Autodesk Inventor part; units mm, degrees
ref_plane "YZ Plane" through (0, 0, 0) normal (1, 0, 0) x (0, 1, 0)
ref_plane "XZ Plane" through (0, 0, 0) normal (0, 1, 0) x (-1, 0, 0)
ref_plane "XY Plane" through (0, 0, 0) normal (0, 0, 1) x (1, 0, 0)
sketch "Sketch1" plane through (0, 0, 0) normal (0, 0, 1) x (1, 0, 0)
  line L0 (29.994, -18.6437) -> (-29.994, -18.6437)
  line L1 (-29.994, 18.6437) -> (29.994, 18.6437)
  line L2 (29.994, -18.6437) -> (-29.994, 18.6437) construction
  line L3 (-29.994, -18.6437) -> (29.994, 18.6437) construction
  line L4 (29.994, -18.6437) -> (-29.994, -18.6437)
  line L5 (-29.994, -18.6437) -> (-29.994, -17.0588)
  line L6 (-29.994, -17.0588) -> (29.994, -17.0588)
  line L7 (29.994, -17.0588) -> (29.994, -18.6437)
  line L8 (-29.994, 18.6437) -> (-29.994, -17.0588)
  line L9 (29.994, 18.6437) -> (29.994, -17.0588)
  point P0 (0, 0)
extrude "Extrusion1" add sketch "Sketch1" against normal blind 1.5875 contours L6 L8 L1 L9
extrude "Extrusion2" add sketch "Sketch1" along normal blind 11.9062 and the other way blind 1.5875 contours L0 L5 L6 L7
sketch "Sketch2" plane through (-29.994, -17.0588, 0) normal (0, 1, 0) x (1, 0, 0)
  circle A0 centre (4.7625, -5.9531) radius 2.1855
  circle A1 centre (55.5625, -5.9531) radius 2.1855
  point P0 (29.994, 0)
  point P1 (0, 0)
sketch "Sketch3" plane through (0, 0, 0) normal (0, 0, 1) x (1, 0, 0)
  circle A0 centre (-15.2797, 0) radius 2.7871
  circle A1 centre (15.2797, 0) radius 2.7871
extrude "Extrusion3" cut sketch "Sketch3" against normal blind 25.4
extrude "Extrusion4" cut sketch "Sketch2" against normal blind 25.4
fillet "Fillet1" radius 1.5875 1 edges at (0, -18.6437, -1.5875)
properties part number "balun_support"
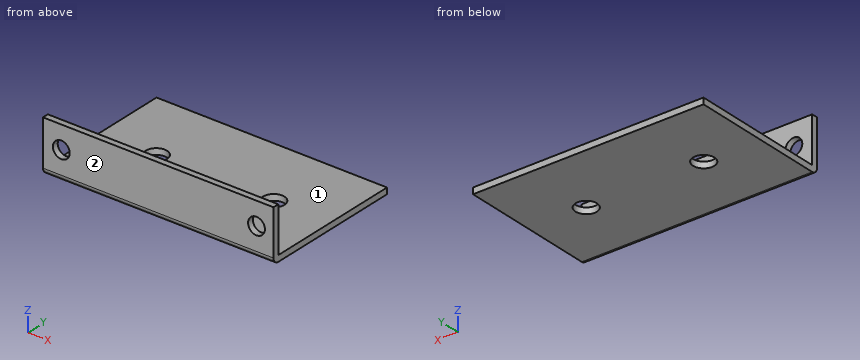
The model under review builds one solid part; all positions refer to its coordinate system, in mm. Face numbers are marked on the shaded views. A direction names the side the tool comes from. Round coordinates to 2 decimals unless told otherwise and drop trailing zeros. Loops run counter-clockwise (first coordinate to the right, second up) from the corner with the lowest first, then second, coordinate; pieces in that order, holes last. Notation, with made-up numbers: (24, 67.5) -> (52, 67.5) arc R20 cw to (52, 94.5) -> close; hole circle Ø8 at (14.5, -10.5). An arc over 180 degrees is marked (long way). Answer as CSV lines item,"result".
1) Add section C-C on z = 7. Write out the cut boundary in (x, y).
Geometry results:
outline,"(-29.99, -18.64) -> (-27.15, -18.64) -> (-27.15, -17.06) -> (-29.99, -17.06) -> close; (-23.31, -18.64) -> (23.65, -18.64) -> (23.65, -17.06) -> (-23.31, -17.06) -> close; (27.49, -18.64) -> (29.99, -18.64) -> (29.99, -17.06) -> (27.49, -17.06) -> close"
2) Add section A-A on y = 0. Write out the cut boundary in (x, z).
Geometry results:
outline,"(-29.99, -1.59) -> (-18.07, -1.59) -> (-18.07, 0) -> (-29.99, 0) -> close; (-12.49, -1.59) -> (12.49, -1.59) -> (12.49, 0) -> (-12.49, 0) -> close; (18.07, -1.59) -> (29.99, -1.59) -> (29.99, 0) -> (18.07, 0) -> close"
3) To check wall thickness, follow line 1 along Y through (x, z) = (-3, 10.25); line 2 along Z through (x, y) = (-10.5, 10). State the ranges of each line that lie inside material, in increasing order. Write a range as from..to.
Geometry results:
line 1,"y = -18.64..-17.06"
line 2,"z = -1.59..0"
4) Add section B-B on x = -13.5. Write out the cut boundary in (y, z) (1 decimal).
Geometry results:
outline,"(-18.6, 0) arc R1.6 ccw to (-17.1, -1.6) -> (-2.1, -1.6) -> (-2.1, 0) -> (-17.1, 0) -> (-17.1, 11.9) -> (-18.6, 11.9) -> close; (2.1, -1.6) -> (18.6, -1.6) -> (18.6, 0) -> (2.1, 0) -> close"
5) Tool access review of the marked faces 1 and 2: name each direction out of +Z, -Z, +X, -X, +Y, -Y from which nothing blocks a thin tool from reaching the whole face with its end or side.
Geometry results:
face 1,"+Z, +X, -X, +Y"
face 2,"+Z, -Z, +X, -X, -Y"
6) Add section D-D on x = 22. Write out the cut boundary in (y, z) (1 decimal), plus the area to 3 significant figures.
Geometry results:
outline,"(-18.6, 0) arc R1.6 ccw to (-17.1, -1.6) -> (18.6, -1.6) -> (18.6, 0) -> (-17.1, 0) -> (-17.1, 11.9) -> (-18.6, 11.9) -> close"
area,"77.5 mm²"
7) For P1, Ø2, axis at x = -6, y = -4.5, coming from the +Z side; P2, Ø5, axis at x = -25.23, z = 5.95, coming from the +Y side, all flat-tipped, find the tip position at first contact; note any pin that passes through.
Geometry results:
P1,"stops at z = 0"
P2,"stops at y = -17.06"
